Can you work these out from the drawing? Everything is in mm from the part's minimum corner. A direction names the side the tool comes from. Give positions to 0.01 mm unless a question says otherwise; leave off trailing zeros. Order: outer loops, then holes, each group sorted by start corner. A loop starts at its lowest first (then second) coordinate and runs counter-clockwise, first axis right, second up. Notation, with made-up numbers: (-17, 81) - (34, 81) arc R14 cw to (34, 105) - close; hole circle Ø11 at (3.5, 3.5). An arc over 180 degrees is marked (long way). Answer as a JSON object with one key per item and string values.
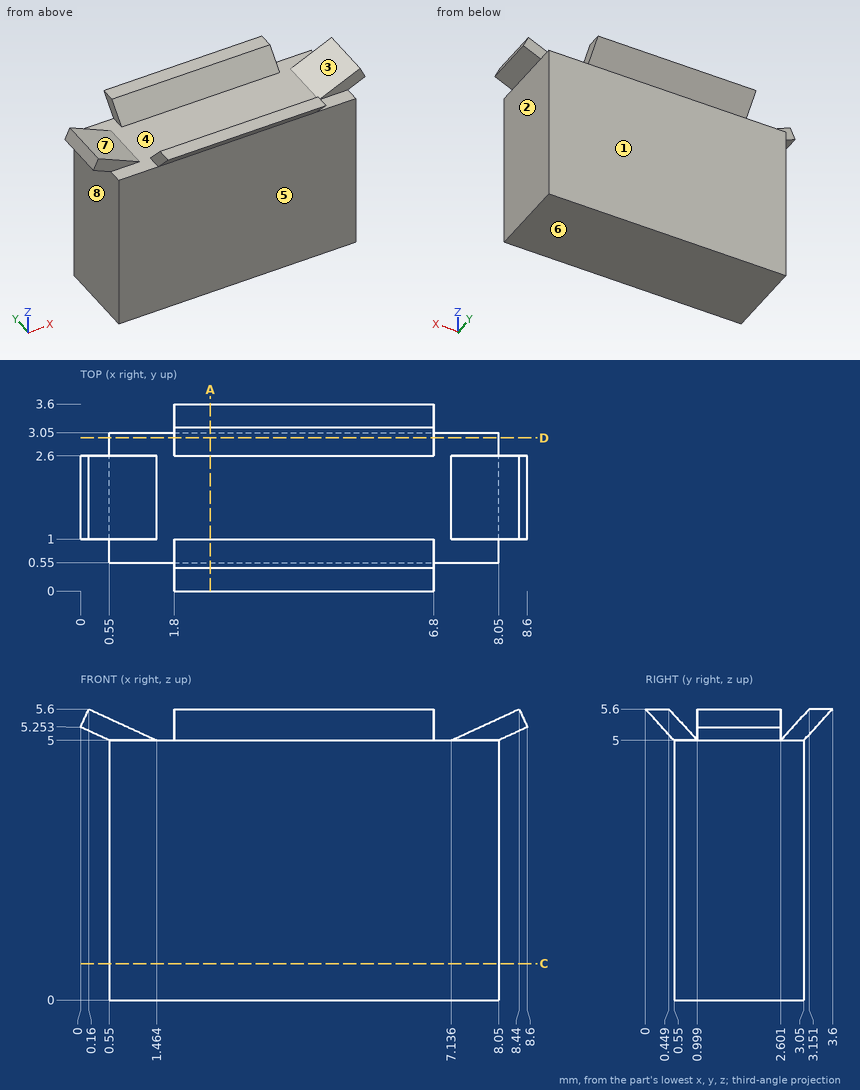
Q1. If we section it at A-A, the plane x = 2.5: Please give me the cut outline in (y, z).
Recorded:
{"outline": "(0, 5.6) - (0.55, 5) - (0.55, 0) - (3.05, 0) - (3.05, 5) - (3.6, 5.6) - (3.15, 5.6) - (2.6, 5) - (1, 5) - (0.45, 5.6) - close"}
Q2. I'm going to push flat-ended pins straight in: pin 1 Ø3 at (x, z) = (6, 2.5) entering from +Y; pin 2 Ø0.5 at (x, z) = (8, 5.5) entering from -Y; pin 3 Ø1.5 at (x, z) = (4, 2.5) entering from -Y. Where does each tip first touch, or does it pass through?
Recorded:
{"pin 1": "stops at y = 3.05", "pin 2": "stops at y = 1", "pin 3": "stops at y = 0.55"}
Q3. We'd pull the mould along X, two halves only. Please class the marked faces 1, 2, 3 and 4: released by +X, released by -X, zero draft, split by the parting line, or undercut.
Recorded:
{"face 1": "zero draft", "face 2": "released by +X", "face 3": "undercut", "face 4": "undercut"}
Q4. If we section it at D-D, the plane y = 2.95: Please give me the cut outline in (x, z).
Recorded:
{"outline": "(0.55, 0) - (8.05, 0) - (8.05, 5) - (6.8, 5) - (6.8, 5.38) - (1.8, 5.38) - (1.8, 5) - (0.55, 5) - close"}
Q5. Which directions (+Z, -Z, +X, -X, +Y, -Y) give clear straight access to the entire face, cutting with the end or side of a thin tool? Please do the marked faces 5, 6, 7 and 8.
Recorded:
{"face 5": "-Z, +X, -X, -Y", "face 6": "-Z, +X, -X, +Y, -Y", "face 7": "+Z, +Y, -Y", "face 8": "-Z, -X, +Y, -Y"}
Q6. I need wall thicknesses on L1, parallel to X at y = 1.05, z = 1.75; L2, parallel to Y at x = 1, z = 4.7; L3, parallel to Z at x = 6, y = 1.2. Which ranges of each line are inside material? Lowest first, please.
Recorded:
{"L1": "x = 0.55 to 8.05", "L2": "y = 0.55 to 3.05", "L3": "z = 0 to 5"}
Q7. If we section it at C-C, the plane z = 0.7: Please give me the cut outline in (x, y).
Recorded:
{"outline": "(0.55, 0.55) - (8.05, 0.55) - (8.05, 3.05) - (0.55, 3.05) - close"}
